```python
from build123d import *

# Parameters (mm, degrees)
SKETCH1_W           = 27.99800038
SKETCH1_H           = 4.5
BOSS_EXTRUDE2_DEPTH = 15
SKETCH2_W           = 27.99800038
SKETCH2_H           = 5
BOSS_EXTRUDE3_DEPTH = 52.81000038
FILLET1_R           = 4
SKETCH3_W           = 27.99800038
SKETCH3_H           = 5
BOSS_EXTRUDE4_DEPTH = 2.000000002
FILLET2_R           = 4
SKETCH4_W           = 3.06400013
SKETCH4_H           = 3.062000231
SKETCH4_W_2         = 3.062003374
BOSS_EXTRUDE5_DEPTH = 6.5
SKETCH5_W           = 12
SKETCH5_H           = 21
CUT_EXTRUDE1_DEPTH  = 6.5
SKETCH6_W           = 3
SKETCH6_H           = 21
BOSS_EXTRUDE6_DEPTH = 12.2
CUT_EXTRUDE2_DEPTH  = 12.2
FILLET4_R           = 3
FILLET5_R           = 3


with BuildPart() as part:
    # Sketch1 → Boss-Extrude2 (new body)
    with BuildSketch(Plane(origin=(0, 0, 0), x_dir=(1, 0, 0), z_dir=(0, 1, 0))):
        with Locations((13.99900019, 2.25)):
            Rectangle(SKETCH1_W, SKETCH1_H)
    extrude(amount=BOSS_EXTRUDE2_DEPTH)

    # Sketch2 → Boss-Extrude3 (add)
    with BuildSketch(Plane.XY):
        with Locations((13.99900019, 2.5)):
            Rectangle(SKETCH2_W, SKETCH2_H)
    extrude(amount=BOSS_EXTRUDE3_DEPTH)

    # Fillet1
    fillet1_edges = [part.edges().sort_by_distance(p)[0] for p in [
        (13.99900019, 5, 0),
    ]]
    fillet(fillet1_edges, radius=FILLET1_R)

    # Sketch3 → Boss-Extrude4 (add)
    with BuildSketch(Plane.XY.offset(52.81000038)):
        Polygon((0, 5), (27.99800038, 5), (27.99800038, 28), (26.52400061, 28), (26.52400061, 26.06971172), (1.52400061, 26.06971172), (1.52400061, 28), (0, 28), align=None)
        with Locations((13.99900019, 2.5)):
            Rectangle(SKETCH3_W, SKETCH3_H)
    extrude(amount=BOSS_EXTRUDE4_DEPTH)

    # Fillet2
    fillet2_edges = [part.edges().sort_by_distance(p)[0] for p in [
        (13.99900019, 5, 52.81000038),
    ]]
    fillet(fillet2_edges, radius=FILLET2_R)

    # Sketch4 → Boss-Extrude5 (add)
    with BuildSketch(Plane(origin=(0, 15, 0), x_dir=(1, 0, 0), z_dir=(0, 1, 0))):
        with Locations((22.327996787, 1.728999914)):
            Rectangle(SKETCH4_W, SKETCH4_H)
        with Locations((4.258997735, 1.728999914)):
            Rectangle(SKETCH4_W_2, SKETCH4_H)
    extrude(amount=BOSS_EXTRUDE5_DEPTH)

    # Sketch5 → Cut-Extrude1 (cut)
    with BuildSketch(Plane.XZ):
        with Locations((13.99800038, 32.310000382)):
            Rectangle(SKETCH5_W, SKETCH5_H)
    extrude(amount=-CUT_EXTRUDE1_DEPTH, mode=Mode.SUBTRACT)

    # Sketch6 → Boss-Extrude6 (add)
    with BuildSketch(Plane.XZ):
        with Locations((6.49800038, 32.310000382)):
            Rectangle(SKETCH6_W, SKETCH6_H)
    extrude(amount=BOSS_EXTRUDE6_DEPTH)

    # Sketch7 → Cut-Extrude2 (cut)
    with BuildSketch(Plane.ZY.offset(-4.99800038)):
        with BuildLine():
            ThreePointArc((24.810000382, -7.65), (23.260000382, -9.2), (24.810000382, -10.75))
            ThreePointArc((24.810000382, -10.75), (26.360000382, -9.2), (24.810000382, -7.65))
        make_face()
        with BuildLine():
            ThreePointArc((39.810000382, -7.65), (38.260000382, -9.2), (39.810000382, -10.75))
            ThreePointArc((39.810000382, -10.75), (41.360000382, -9.2), (39.810000382, -7.65))
        make_face()
    extrude(amount=-CUT_EXTRUDE2_DEPTH, mode=Mode.SUBTRACT)

    # Fillet4
    fillet4_edges = [part.edges().sort_by_distance(p)[0] for p in [
        (6.49800038, -12.2, 42.810000382),
        (6.49800038, -12.2, 21.810000382),
    ]]
    fillet(fillet4_edges, radius=FILLET4_R)

    # Fillet5
    fillet5_edges = [part.edges().sort_by_distance(p)[0] for p in [
        (6.49800038, 0, 42.810000382),
        (6.49800038, 0, 21.810000382),
    ]]
    fillet(fillet5_edges, radius=FILLET5_R)


solid = part.part
```
Part model, mm, in its own coordinate system. A direction names the side the tool comes from. Round coordinates to 2 decimals unless told otherwise and drop trailing zeros. Loops run counter-clockwise (first coordinate to the right, second up) from the corner with the lowest first, then second, coordinate; pieces in that order, holes last.
1. Flat gauge pins, fed straight in: pin 1 (1.5 mm diameter, centred on x = 10.5, z = 44.5, fed in from -Y); pin 2 (3.5 mm diameter, centred on y = 18, z = -1.5, fed in from -X); pin 3 (0.9 mm diameter, centred on x = 6.5, y = -4.5, fed in from -Z). Where does each tip first touch, or does it go through?
Solutions:
pin 1: stops at y = 0
pin 2: stops at x = 2.73
pin 3: stops at z = 21.81
2. Slice it at D-D (y = -8.5). Give the cut face in (x, z).
Solutions:
outline: (5, 21.81) - (8, 21.81) - (8, 23.43) - (5, 23.43) - close; (5, 26.19) - (8, 26.19) - (8, 38.43) - (5, 38.43) - close; (5, 41.19) - (8, 41.19) - (8, 42.81) - (5, 42.81) - close
3. Drill centre lines: line 1 along Z through (x, y) = (6.4, -9.2); line 2 along X through (y, z) = (-6.5, 28); line 3 along Y through (x, z) = (13.75, 14). Where is each one in solid material? Low to high.
Solutions:
line 1: z = 21.81 to 23.26, 26.36 to 38.26, 41.36 to 42.81
line 2: x = 5 to 8
line 3: y = 0 to 5
4. Slice it at A-A (z = 35). Give the cut face in (x, y), and give its area (3 significant figures).
Solutions:
outline: (0, 0) - (5, 0) - (5, -12.2) - (8, -12.2) - (8, 5) - (0, 5) - close; (20, 0) - (28, 0) - (28, 5) - (20, 5) - close
area: 117 mm2
5. 3-axis set-ups, long thin cutter, end or side, ignore diameter. For faces 4 (the face through (4, 18, -3.26)), 5 (the face through (14, 5, 21)), 6 (the face through (6, -6, 21.81)), 7 (the face through (1.524, 27, 54)): which of +Z, -Z, +X, -X, +Y, -Y reach the whole face in a straight line?
Solutions:
face 4: -Z, +X, -X, +Y
face 5: +X, -X, +Y
face 6: -Z, +X, -X, -Y
face 7: +Z, -Z, +Y
6. Slice it at C-C (x = 9.5). Give the cut face in (y, z), and give its area (3 significant figures).
Solutions:
outline: (0, -4.5) - (15, -4.5) - (15, 0) - (9, 0) arc R4 cw to (5, 4) - (5, 21.81) - (0, 21.81) - close; (0, 42.81) - (5, 42.81) - (5, 48.81) arc R4 cw to (9, 52.81) - (26.07, 52.81) - (26.07, 54.81) - (0, 54.81) - close
area: 286 mm2
7. Slice it at B-B (y = 14). Give the cut face in (x, z), and give its area (3 significant figures).
Solutions:
outline: (0, -4.5) - (28, -4.5) - (28, 0) - (0, 0) - close; (0, 52.81) - (28, 52.81) - (28, 54.81) - (0, 54.81) - close
area: 182 mm2
8. Two-plate mould, pull along X, no slides. Class faces 1 (the face through (19.998, 2, 32)), 2 (the face through (6.477, -8.998, 26.347)), 3 (the face through (0, 4.7, 25)): pulls with the +X half, pulls with the -X half, needs draft (parallel to the pull), parting line crosses it, or undercut.
Solutions:
face 1: undercut
face 2: needs draft
face 3: pulls with the -X half
